Build history of the part. All positions in model axes, mm. A direction names the side the tool comes from. Round coordinates to 2 decimals unless told otherwise and drop trailing zeros. Write each loop counter-clockwise with the first axis right and the second up, starting at its lowest first coordinate (ties: lowest second). Pieces come first, ordered by that corner, then holes. Notation, with made-up numbers: M 59.5,0 L 82.5,0 A26 ccw 82.5,17 Z; hole C -30,26.5 d4. An arc over 180 degrees is marked long. Write item = value, one per line.
from build123d import *

# Parameters (mm, degrees)
F2_R     = 71
F2_R_2   = 70
F3_DEPTH = 22
F2_R_3   = 5
F4_DEPTH = 2
F5_R     = 1


with BuildPart() as f3:
    # F2 (on Top) → F3 (new body)
    with BuildSketch(Plane.XY):
        Circle(F2_R)
        Circle(F2_R_2, mode=Mode.SUBTRACT)
    extrude(amount=F3_DEPTH)

    # F2 (on Top) → F4 (join)
    with BuildSketch(Plane.XY):
        Circle(F2_R_2)
        with BuildLine():
            ThreePointArc((62.7851787088, 16.8232379317), (64.4439159893, 8.4842024943), (65, 0))
            ThreePointArc((65, 0), (8.4842024943, -64.4439159893), (-62.7851787088, -16.8232379317))
            ThreePointArc((-62.7851787088, -16.8232379317), (-64.4439159893, -8.4842024943), (-65, 0))
            ThreePointArc((-65, 0), (-8.4842024943, 64.4439159893), (62.7851787088, 16.8232379317))
        make_face(mode=Mode.SUBTRACT)
        with BuildLine():
            ThreePointArc((-53.1259204459, -14.2350474806), (7.1789405721, -54.5294673756), (55, 0))
            ThreePointArc((55, 0), (54.5294673756, 7.1789405721), (53.1259204459, 14.2350474806))
            ThreePointArc((53.1259204459, 14.2350474806), (-7.1789405721, 54.5294673756), (-55, 0))
            ThreePointArc((-55, 0), (-54.5294673756, -7.1789405721), (-53.1259204459, -14.2350474806))
        make_face()
        with BuildLine():
            ThreePointArc((17.1010071663, 46.9846310393), (40.9576022144, 28.6788218176), (50, 0))
            ThreePointArc((50, 0), (35.3553390593, -35.3553390593), (0, -50))
            ThreePointArc((0, -50), (-8.6824088833, -49.2403876506), (-17.1010071663, -46.9846310393))
            ThreePointArc((-17.1010071663, -46.9846310393), (-49.2403876506, 8.6824088833), (0, 50))
            ThreePointArc((0, 50), (8.6824088833, 49.2403876506), (17.1010071663, 46.9846310393))
        make_face(mode=Mode.SUBTRACT)
        with BuildLine():
            ThreePointArc((40, 0), (32.7660817716, 22.943057454), (13.680805733, 37.5877048314))
            ThreePointArc((13.680805733, 37.5877048314), (6.9459271067, 39.3923101205), (0, 40))
            ThreePointArc((0, 40), (-39.3923101205, 6.9459271067), (-13.680805733, -37.5877048314))
            ThreePointArc((-13.680805733, -37.5877048314), (-6.9459271067, -39.3923101205), (0, -40))
            ThreePointArc((0, -40), (28.2842712475, -28.2842712475), (40, 0))
        make_face()
        with BuildLine():
            ThreePointArc((32.8892417275, 11.9707050164), (34.4682713554, 6.0776862183), (35, 0))
            ThreePointArc((35, 0), (6.0776862183, -34.4682713554), (-32.8892417275, -11.9707050164))
            ThreePointArc((-32.8892417275, -11.9707050164), (-34.4682713554, -6.0776862183), (-35, 0))
            ThreePointArc((-35, 0), (-6.0776862183, 34.4682713554), (32.8892417275, 11.9707050164))
        make_face(mode=Mode.SUBTRACT)
        with BuildLine():
            ThreePointArc((-23.4923155196, -8.5505035831), (4.3412044417, -24.6201938253), (25, 0))
            ThreePointArc((25, 0), (24.6201938253, 4.3412044417), (23.4923155196, 8.5505035831))
            ThreePointArc((23.4923155196, 8.5505035831), (-4.3412044417, 24.6201938253), (-25, 0))
            ThreePointArc((-25, 0), (-24.6201938253, -4.3412044417), (-23.4923155196, -8.5505035831))
        make_face()
        Circle(F2_R_3, mode=Mode.SUBTRACT)
        with BuildLine():
            ThreePointArc((-17.1010071663, -46.9846310393), (-8.6824088833, -49.2403876506), (0, -50))
            Line((0, -50), (0, -40))
            ThreePointArc((0, -40), (-6.9459271067, -39.3923101205), (-13.680805733, -37.5877048314))
            Line((-13.680805733, -37.5877048314), (-17.1010071663, -46.9846310393))
        make_face()
        with BuildLine():
            Line((13.680805733, 37.5877048314), (17.1010071663, 46.9846310393))
            ThreePointArc((17.1010071663, 46.9846310393), (8.6824088833, 49.2403876506), (0, 50))
            Line((0, 50), (0, 40))
            ThreePointArc((0, 40), (6.9459271067, 39.3923101205), (13.680805733, 37.5877048314))
        make_face()
        with BuildLine():
            ThreePointArc((-65, 0), (-64.4439159893, -8.4842024943), (-62.7851787088, -16.8232379317))
            Line((-62.7851787088, -16.8232379317), (-53.1259204459, -14.2350474806))
            ThreePointArc((-53.1259204459, -14.2350474806), (-54.5294673756, -7.1789405721), (-55, 0))
            Line((-55, 0), (-65, 0))
        make_face()
        with BuildLine():
            Line((55, 0), (65, 0))
            ThreePointArc((65, 0), (64.4439159893, 8.4842024943), (62.7851787088, 16.8232379317))
            Line((62.7851787088, 16.8232379317), (53.1259204459, 14.2350474806))
            ThreePointArc((53.1259204459, 14.2350474806), (54.5294673756, 7.1789405721), (55, 0))
        make_face()
        with BuildLine():
            ThreePointArc((-35, 0), (-34.4682713554, -6.0776862183), (-32.8892417275, -11.9707050164))
            Line((-32.8892417275, -11.9707050164), (-23.4923155196, -8.5505035831))
            ThreePointArc((-23.4923155196, -8.5505035831), (-24.6201938253, -4.3412044417), (-25, 0))
            Line((-25, 0), (-35, 0))
        make_face()
        with BuildLine():
            Line((25, 0), (35, 0))
            ThreePointArc((35, 0), (34.4682713554, 6.0776862183), (32.8892417275, 11.9707050164))
            Line((32.8892417275, 11.9707050164), (23.4923155196, 8.5505035831))
            ThreePointArc((23.4923155196, 8.5505035831), (24.6201938253, 4.3412044417), (25, 0))
        make_face()
    extrude(amount=F4_DEPTH)

    # F5
    f5_edges = [f3.edges().sort_by_distance(p)[0] for p in [
        (-71, 0, 0),
    ]]
    fillet(f5_edges, radius=F5_R)


solid = f3.part
1. Band-saw the part on B-B (y = 22.5). Count the separate pieces of the cut face and the enclosed holes in it, plus the area to 3 significant figures.
Responses:
separate_pieces = 7
enclosed_holes = 0
area = 158 mm²
2. Band-saw the part on A-A (z = 15.5). List the corners of the cut face in (x, y), plus the area to 3 significant figures.
Responses:
outline = C 0,0 d142; hole C 0,0 d140
area = 443 mm²
3. Tool access for faces 1 (the face through (-1, -15, 0)), 2 (the face through (9.78, -64.26, 0.99)), 3 (the face through (-1, -15, 2)): list every direction of +Z, -Z, +X, -X, +Y, -Y with a clear straight run to the whole face (end or side of a thin tool).
Responses:
face_1 = -Z, +X, -X, +Y, -Y
face_2 = +Z, -Z
face_3 = +Z
4. Probe probe 1 along Y at (x, z) = (0, 7); probe 2 along X at (y, z) = (-42.5, 19); probe 3 along X at (y, z) = (-58.5, 20.5). List the from-to ranges inside material, lowest first.
Responses:
probe_1 = -71 to -70, 70 to 71
probe_2 = -56.87 to -55.62, 55.62 to 56.87
probe_3 = -40.23 to -38.44, 38.44 to 40.23
5. Mould opens along X. For faces 4 (the face through (-15.39, -69.31, 11.35)), 5 (the face through (6.75, -34.343, 0.986)), 6 (the face through (52.3, -47, 22)) say: pulls with the +X half, pulls with the -X half, needs draft (parallel to the pull), parting line crosses it, or undercut.
Responses:
face_4 = parting line crosses it
face_5 = undercut
face_6 = needs draft
6. Flat gauge pins, fed straight in: pin 1 (8 mm diameter, centred on x = 0, y = 0, fed in from -Z); pin 2 (2 mm diameter, centred on x = 32, z = 0.5, fed in from -Y); pin 3 (0.6 mm diameter, centred on y = -47.5, z = 1, fed in from +X); pin 4 (3 mm diameter, centred on y = 29, z = 6, fed in from +X). Where does each tip first touch, or does it go through?
Responses:
pin_1 = through
pin_2 = -63.83
pin_3 = 53.04
pin_4 = 65.46
